```python
from build123d import *

# Parameters (mm, degrees)
SKETCH_1_R          = 1.85
EXTRUDE_1_DEPTH     = 13
SKETCH_2_R          = 2.6
CUT_EXTRUDE_1_DEPTH = 10
SKETCH_3_R          = 2.6
CUT_EXTRUDE_2_DEPTH = 10
FILLET_1_R          = 2
FILLET_2_R          = 1
SKETCH_4_R          = 3.5
SKETCH_4_R_2        = 1.85
CUT_EXTRUDE_3_DEPTH = 7
CUT_EXTRUDE_5_DEPTH = 61.729236251
CUT_EXTRUDE_START   = -4
SKETCH_6_R          = 5.5
SKETCH_6_R_2        = 2.6
CUT_EXTRUDE_6_DEPTH = 4
SKETCH_7_R          = 5.5
SKETCH_7_R_2        = 2.6
CUT_EXTRUDE_7_DEPTH = 4
SKETCH_8_R          = 35.1
CUT_EXTRUDE_8_DEPTH = 61.729236251


with BuildPart() as part:
    # 草图1 → 凸台-拉伸1 (new body)
    with BuildSketch(Plane(origin=(0, 0, 0), x_dir=(1, 0, 0), z_dir=(0, 1, 0))):
        with BuildLine():
            ThreePointArc((-17.962748608, -30.038969064), (-22.702483698, -26.638266346), (-26.811555509, -22.497566339))
            Line((-26.811555509, -22.497566339), (-36.387111048, -30.53241146))
            ThreePointArc((-36.387111048, -30.53241146), (0, -47.5), (36.387111048, -30.53241146))
            Line((36.387111048, -30.53241146), (26.811555509, -22.497566339))
            ThreePointArc((26.811555509, -22.497566339), (22.702483698, -26.638266346), (17.962748608, -30.038969064))
            Line((17.962748608, -30.038969064), (19.330292732, -33.340512637))
            Line((19.330292732, -33.340512637), (9.906721501, -37.243883647))
            Line((9.906721501, -37.243883647), (8.539177376, -33.942340075))
            ThreePointArc((8.539177376, -33.942340075), (0, -35), (-8.539177376, -33.942340075))
            Line((-8.539177376, -33.942340075), (-9.906721501, -37.243883647))
            Line((-9.906721501, -37.243883647), (-19.330292732, -33.340512637))
            Line((-19.330292732, -33.340512637), (-17.962748608, -30.038969064))
        make_face()
        with BuildLine():
            ThreePointArc((-28.2020382, -30.0520382), (-28.237585432, -30.412955296), (-28.342861065, -30.76000255))
            ThreePointArc((-28.342861065, -30.76000255), (-31.866490969, -29.691121105), (-28.2020382, -30.0520382))
        make_face(mode=Mode.SUBTRACT)
        with BuildLine():
            ThreePointArc((1.85, -42.5), (-0.360917096, -44.314452769), (-1.709177135, -41.79203565))
            ThreePointArc((-1.709177135, -41.79203565), (0.360917096, -40.685547231), (1.85, -42.5))
        make_face(mode=Mode.SUBTRACT)
        with Locations(Location((30.0520382, -30.0520382, 0), (0, 0, 90))):
            Circle(SKETCH_1_R, mode=Mode.SUBTRACT)
    extrude(amount=EXTRUDE_1_DEPTH)

    # 草图2 → 切除-拉伸1 (cut)
    with BuildSketch(Plane(origin=(-14.618507116, 0, 35.292198142), x_dir=(-0.9238795325112864, 0, -0.38268343236509067), z_dir=(0.38268343236509067, 0, -0.9238795325112864))):
        with Locations((0, 6.5)):
            Circle(SKETCH_2_R)
    extrude(amount=-CUT_EXTRUDE_1_DEPTH, mode=Mode.SUBTRACT)

    # 草图3 → 切除-拉伸2 (cut)
    with BuildSketch(Plane(origin=(14.618507116, 0, 35.292198142), x_dir=(-0.9238795325112864, 0, 0.38268343236509067), z_dir=(-0.38268343236509067, 0, -0.9238795325112864))):
        with Locations((0, 6.5)):
            Circle(SKETCH_3_R)
    extrude(amount=-CUT_EXTRUDE_2_DEPTH, mode=Mode.SUBTRACT)

    # 圆角1
    fillet_1_edges = [part.edges().sort_by_distance(p)[0] for p in [
        (-26.811555509, 6.5, 22.497566339),
        (26.811555509, 6.5, 22.497566339),
        (36.387111048, 6.5, 30.53241146),
        (-36.387111048, 6.5, 30.53241146),
    ]]
    fillet(fillet_1_edges, radius=FILLET_1_R)

    # 圆角2
    fillet_2_edges = [part.edges().sort_by_distance(p)[0] for p in [
        (-17.962748608, 6.5, 30.038969064),
        (-8.539177376, 6.5, 33.942340075),
        (8.539177376, 6.5, 33.942340075),
        (17.962748608, 6.5, 30.038969064),
    ]]
    fillet(fillet_2_edges, radius=FILLET_2_R)

    # 草图4 → 切除-拉伸3 (cut)
    # profile 1 of 3: a face of its own
    with BuildSketch(Plane.XZ):
        with Locations(Location((-30.0520382, 30.0520382, 0), (0, 0, 270))):
            Circle(SKETCH_4_R)
        with Locations(Location((-30.0520382, 30.0520382, 0), (0, 0, 270))):
            Circle(SKETCH_4_R_2, mode=Mode.SUBTRACT)
    # profile 2 of 3: a face of its own
    with BuildSketch(Plane.XZ):
        with Locations(Location((0, 42.5, 0), (0, 0, 270))):
            Circle(SKETCH_4_R)
        with Locations(Location((0, 42.5, 0), (0, 0, 270))):
            Circle(SKETCH_4_R_2, mode=Mode.SUBTRACT)
    # profile 3 of 3: a face of its own
    with BuildSketch(Plane.XZ):
        with Locations(Location((30.0520382, 30.0520382, 0), (0, 0, 270))):
            Circle(SKETCH_4_R)
        with Locations(Location((30.0520382, 30.0520382, 0), (0, 0, 270))):
            Circle(SKETCH_4_R_2, mode=Mode.SUBTRACT)
    extrude(amount=-CUT_EXTRUDE_3_DEPTH, mode=Mode.SUBTRACT)

    # 草图5 → 切除-拉伸5 (cut, through all)
    with BuildSketch(Plane.XZ):
        with BuildLine():
            Line((-22.784170244, 41.67891057), (-18.072384629, 43.630596075))
            Line((-18.072384629, 43.630596075), (-18.177463037, 43.884277794))
            ThreePointArc((-18.177463037, 43.884277794), (-20.510479308, 42.843555391), (-22.784170244, 41.67891057))
        make_face()
        with BuildLine():
            Line((-18.177463037, 43.884277794), (-18.072384629, 43.630596075))
            Line((-18.072384629, 43.630596075), (-13.360599013, 45.58228158))
            ThreePointArc((-13.360599013, 45.58228158), (-15.791869544, 44.798067551), (-18.177463037, 43.884277794))
        make_face()
        with BuildLine():
            ThreePointArc((18.177463037, 43.884277794), (15.791869544, 44.798067551), (13.360599013, 45.58228158))
            Line((13.360599013, 45.58228158), (18.072384629, 43.630596075))
            Line((18.072384629, 43.630596075), (18.177463037, 43.884277794))
        make_face()
        with BuildLine():
            Line((18.177463037, 43.884277794), (18.072384629, 43.630596075))
            Line((18.072384629, 43.630596075), (22.784170244, 41.67891057))
            ThreePointArc((22.784170244, 41.67891057), (20.510479308, 42.843555391), (18.177463037, 43.884277794))
        make_face()
    extrude(amount=-CUT_EXTRUDE_5_DEPTH, mode=Mode.SUBTRACT)

    # 草图6 → 切除-拉伸6 (cut)
    with BuildSketch(Plane(origin=(-18.072384629, 0, 43.630596075), x_dir=(0.9238795325112865, 0, 0.38268343236509045), z_dir=(-0.38268343236509045, 0, 0.9238795325112865)).offset(CUT_EXTRUDE_START)):
        with Locations((0, 6.5)):
            Circle(SKETCH_6_R)
        with Locations(Location((0, 6.5, 0), (0, 0, 180))):
            Circle(SKETCH_6_R_2, mode=Mode.SUBTRACT)
    extrude(amount=CUT_EXTRUDE_6_DEPTH, mode=Mode.SUBTRACT)

    # 草图7 → 切除-拉伸7 (cut)
    with BuildSketch(Plane(origin=(18.072384629, 0, 43.630596075), x_dir=(0.9238795325112865, 0, -0.38268343236509045), z_dir=(0.38268343236509045, 0, 0.9238795325112865)).offset(CUT_EXTRUDE_START)):
        with Locations((0, 6.5)):
            Circle(SKETCH_7_R)
        with Locations(Location((0, 6.5, 0), (0, 0, 180))):
            Circle(SKETCH_7_R_2, mode=Mode.SUBTRACT)
    extrude(amount=CUT_EXTRUDE_7_DEPTH, mode=Mode.SUBTRACT)

    # 草图8 → 切除-拉伸8 (cut, through all)
    with BuildSketch(Plane(origin=(0, 13, 0), x_dir=(1, 0, 0), z_dir=(0, 1, 0))):
        Circle(SKETCH_8_R)
    extrude(amount=-CUT_EXTRUDE_8_DEPTH, mode=Mode.SUBTRACT)


solid = part.part
```
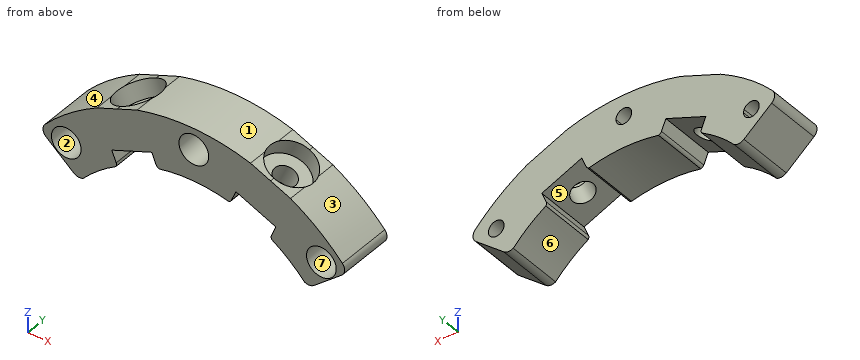
Check sheet for the modelled part. Datum: model origin and axes. Units: mm. Face numbers are marked on the shaded views. A direction names the side the tool comes from. Give positions to 0.01 mm unless a question says otherwise; leave off trailing zeros. Loops run counter-clockwise (first coordinate to the right, second up) from the corner with the lowest first, then second, coordinate; pieces in that order, holes last. Notation, with made-up numbers: (-4.75, -35) - (13.25, -35) arc R13 ccw to (13.25, -14) - close; hole circle Ø7 at (-29, 86). An arc over 180 degrees is marked (long way). One line per question, with ' | ' between items. Start each with the question number.
1. Gauge pin test, flat ends, axial feed: pin 1 Ø4 at (y, z) = (5, 43) entering from -X; pin 2 Ø6 at (x, z) = (30.05, 30.05) entering from -Y; pin 3 Ø1.5 at (x, y) = (-11, 1.5) entering from +Z. Record the tip position at first contact, or that the pin passes through.
2. Draft check along X on the marked faces 1, 2 and 3. Enter one of: released by +X, released by -X, zero draft, split by the parting line, or undercut.
3. Set-up check for the marked faces 4, 5, 6 and 7: record each of +Z, -Z, +X, -X, +Y, -Y from which the full face is reachable in a straight line by a thin tool's end or side.
4. Material ranges on line 1 along X through (y, z) = (11.4, 42.5); line 2 along Z through (x, y) = (0, 10.25); line 3 along X through (y, z) = (6, 32), recorded low to high. Write a range as [from, to].
5. Cross-section at B-B, the plane y = 10. Give the number of separate pieces and of enclosed holes in the cut face, plus the area to 3 significant figures.
6. Cross-section at A-A, the plane x = 0. Enter the section's corners in (y, z).
Check result:
1) pin 1: stops at x = -23.98 | pin 2: stops at y = 7 | pin 3: stops at z = 46.38
2) face 1: split by the parting line | face 2: undercut | face 3: released by +X
3) face 4: +Z, -X, +Y, -Y | face 5: +Y, -Y | face 6: -Z, +Y, -Y | face 7: -Y
4) line 1: x = [-20.8, -20.31], [-14.9, -1.85], [1.85, 14.9], [20.31, 20.8] | line 2: z = [35.1, 40.65], [44.35, 47.5] | line 3: x = [-35.1, -32.96], [-27.14, -18.78], [18.78, 27.14], [32.96, 35.1]
5) separate pieces: 1 | enclosed holes: 3 | area: 721 mm2
6) outline: (0, 35.1) - (13, 35.1) - (13, 40.65) - (7, 40.65) - (7, 39) - (0, 39) - close; (0, 46) - (7, 46) - (7, 44.35) - (13, 44.35) - (13, 47.5) - (0, 47.5) - close
